The model under review builds one solid part; all positions refer to its coordinate system, in mm. A direction names the side the tool comes from. Coordinates: 2 decimals unless noted, no trailing zeros. Write each loop counter-clockwise with the first axis right and the second up, starting at its lowest first coordinate (ties: lowest second). Pieces come first, ordered by that corner, then holes.
1) Add section A-A, the plane x = 16.5. State the section outline as (y, z) points.
2) For P1, Ø1.5, axis at y = 152.5, z = -1, coming from the -X side; P2, Ø1, axis at x = -19, z = -7, coming from the -Y side; P3, Ø0.8, axis at y = 135.5, z = -0.5, coming from the +X side; P4, Ø2.5, axis at x = -24.73, y = 109, coming from the +Z side, all flat-tipped, find the tip position at first contact; note any pin that passes through.
3) Add section C-C, the plane z = -6.25. State the section outline as (x, y) points, then the cut area to 3 significant figures.
4) Add section B-B, the plane y = 44.5. State the section outline as (x, z) points, then the cut area to 3 significant figures.
5) For line 1 (Z direction, x = 31.5, y = 92.5); line 2 (X direction, y = 22, z = -0.25); line 3 (Y direction, x = 29, z = -0.7), list the stretches that pass through material, from the lowest coordinate up.
6) Machinability: for faces 5 (the flat face through (-1, 97, -1)), 6 (the flat face through (35.323, 86.552, -0.493)), 7 (the flat face through (1, 213, -8.485)), 8 (the flat face through (-35.177, 87.448, -0.493)), which of the approach directions +Z, -Z, +X, -X, +Y, -Y give a long, thin tool a straight path to every point of the face, cutting with its end or side? Answer none if there is none.
7) Mouldability with a two-part tool opening along Y and no side actions: class faces 1 (the cylindrical face through (46.996, 159.626, -0.493)), 2 (the flat face through (-1, 97, 0)), 3 (the cylindrical face through (-46.996, 160.374, -0.493)), 4 (the flat face through (-0.42, 196.749, -4.335)) as released by +Y, released by -Y, zero draft, split by the parting line, or undercut.
from build123d import *

# Parameters (mm, degrees)
BASE_FLANGE1_DEPTH           = 1
EDGE_FLANGE1_STRIP_CUT_DEPTH = 60
EDGE_FLANGE1_DEPTH           = 60
EDGE_FLANGE2_STRIP_CUT_DEPTH = 60
EDGE_FLANGE2_DEPTH           = 60
SKETCH14_W                   = 1
SKETCH14_H                   = 24.280676727
BOSS_EXTRUDE1_DEPTH          = 9
SKETCH15_W                   = 1
SKETCH15_H                   = 24.280676727
BOSS_EXTRUDE2_DEPTH          = 9
CUT_EXTRUDE1_START           = -1
CUT_EXTRUDE1_DEPTH           = 1
FILLET2_R                    = 2
SKETCH17_R                   = 1.5
CUT_EXTRUDE2_DEPTH           = 231.487770095
SKETCH18_R                   = 1.5
CUT_EXTRUDE3_DEPTH           = 231.487770095
SKETCH19_R                   = 1.5
CUT_EXTRUDE4_DEPTH           = 231.487770095


# Read off the part's stored shape, not the designer's step: Cut-Extrude1
# Sheet-metal steps are written as plain solids
with BuildPart() as part:
    # Sketch1 → Base-Flange1 (new body)
    with BuildSketch(Plane.XY):
        with BuildLine():
            Line((-40.5, 0), (40.5, 0))
            Line((40.5, 0), (40.5, 55))
            Line((40.5, 55), (30, 119))
            Line((30, 119), (30, 143))
            ThreePointArc((30, 143), (47, 160), (30, 177))
            Line((30, 177), (30, 192))
            Line((30, 192), (-30, 192))
            Line((-30, 192), (-30, 177))
            ThreePointArc((-30, 177), (-47, 160), (-30, 143))
            Line((-30, 143), (-30, 119))
            Line((-30, 119), (-40.5, 55))
            Line((-40.5, 55), (-40.5, 0))
        make_face()
    extrude(amount=-BASE_FLANGE1_DEPTH)

    # Edge-Flange1 strip (across the edge) → Edge-Flange1 strip cut (cut)
    with BuildSketch(Plane(origin=(-30, 192, -1), x_dir=(0, -0.7071067811865438, -0.7071067811865512), z_dir=(1, 0, 0))):
        Polygon((-4.361498471, 2.947284909), (-0.491361636, -0.922851926), (0.215745145, -0.215745145), (-3.65439169, 3.65439169), align=None)
    extrude(amount=EDGE_FLANGE1_STRIP_CUT_DEPTH, mode=Mode.SUBTRACT)

    # Edge-Flange1 section (across the edge) → Edge-Flange1 (add)
    with BuildSketch(Plane(origin=(-30, 192, -1), x_dir=(0, -0.7071067811865438, -0.7071067811865512), z_dir=(1, 0, 0))):
        with BuildLine():
            Line((-1, 0.30510971), (-1, 11.585786438))
            Line((-1, 11.585786438), (0, 11.585786438))
            Line((0, 11.585786438), (0, 0.30510971))
            ThreePointArc((0, 0.30510971), (0.056070336, 0.023225094), (0.215745145, -0.215745145))
            Line((0.215745145, -0.215745145), (-0.491361636, -0.922851926))
            ThreePointArc((-0.491361636, -0.922851926), (-0.867809196, -0.359458339), (-1, 0.30510971))
        make_face()
    extrude(amount=EDGE_FLANGE1_DEPTH)

    # Edge-Flange2 strip (across the edge) → Edge-Flange2 strip cut (cut)
    with BuildSketch(Plane(origin=(30, 200.899494937, -8.485281374), x_dir=(0, 0, 1), z_dir=(-1, 0, 0))):
        Polygon((-4.361498471, 2.947284909), (-0.491361636, -0.922851926), (0.215745145, -0.215745145), (-3.65439169, 3.65439169), align=None)
    extrude(amount=EDGE_FLANGE2_STRIP_CUT_DEPTH, mode=Mode.SUBTRACT)

    # Edge-Flange2 section (across the edge) → Edge-Flange2 (add)
    with BuildSketch(Plane(origin=(30, 200.899494937, -8.485281374), x_dir=(0, 0, 1), z_dir=(-1, 0, 0))):
        with BuildLine():
            Line((-1, 0.30510971), (-1, 24.585786438))
            Line((-1, 24.585786438), (0, 24.585786438))
            Line((0, 24.585786438), (0, 0.30510971))
            ThreePointArc((0, 0.30510971), (0.056070336, 0.023225094), (0.215745145, -0.215745145))
            Line((0.215745145, -0.215745145), (-0.491361636, -0.922851926))
            ThreePointArc((-0.491361636, -0.922851926), (-0.867809196, -0.359458339), (-1, 0.30510971))
        make_face()
    extrude(amount=EDGE_FLANGE2_DEPTH)

    # Sketch14 → Boss-Extrude1 (add)
    with BuildSketch(Plane(origin=(30, 0, 0), x_dir=(0, 0, -1), z_dir=(1, 0, 0))):
        with Locations((8.985281374, 213.344943011)):
            Rectangle(SKETCH14_W, SKETCH14_H)
    extrude(amount=BOSS_EXTRUDE1_DEPTH)

    # Sketch15 → Boss-Extrude2 (add)
    with BuildSketch(Plane.ZY.offset(30)):
        with Locations((-8.985281374, 213.344943011)):
            Rectangle(SKETCH15_W, SKETCH15_H)
    extrude(amount=BOSS_EXTRUDE2_DEPTH)

    # Cut-Extrude1 outline → Cut-Extrude1 (cut)
    with BuildSketch(Plane(origin=(0, 0, -9.485281374), x_dir=(-1, 0, 0), z_dir=(0, 0, -1)).offset(CUT_EXTRUDE1_START)):
        with BuildLine():
            Line((39, 201.204604647), (39, 219.240417061))
            add(Edge.make_bspline(
                [(30, 201.204604647), (31.71398357, 204.270148777), (35.194685688, 209.766177292), (38.784446875, 217.082662856), (39, 219.240417061)],
                knots=[0, 0, 0, 0, 0.463591524, 0.691545034, 0.691545034, 0.691545034, 0.691545034], degree=3))
            Line((30, 201.204604647), (39, 201.204604647))
        make_face()
        with BuildLine():
            add(Edge.make_bspline(
                [(39, 220.550582239), (38.73699137, 222.877809464), (36.937902842, 224.748781209), (32.132158029, 225.485281374)],
                knots=[0.73898762, 0.73898762, 0.73898762, 0.73898762, 1, 1, 1, 1], degree=3))
            Line((39, 220.550582239), (39, 225.485281374))
            Line((39, 225.485281374), (32.132158029, 225.485281374))
        make_face()
    cut_extrude1 = extrude(amount=CUT_EXTRUDE1_DEPTH, mode=Mode.SUBTRACT)

    # Mirror1: Cut-Extrude1 across plane
    add(cut_extrude1.mirror(Plane(origin=(0, 0, 0), x_dir=(0, 0, 1), z_dir=(1, 0, 0))), mode=Mode.SUBTRACT)

    # Fillet2
    fillet2_edges = [part.edges().sort_by_distance(p)[0] for p in [
        (40.5, 0, -0.5),
        (-40.5, 0, -0.5),
    ]]
    fillet(fillet2_edges, radius=FILLET2_R)

    # Sketch17 → Cut-Extrude2 (cut, through all)
    with BuildSketch(Plane(origin=(0, 0, -1), x_dir=(-1, 0, 0), z_dir=(0, 0, -1))):
        with Locations((-35.5, 5)):
            Circle(SKETCH17_R)
        with Locations((35.5, 5)):
            Circle(SKETCH17_R)
        with Locations((-35.5, 55)):
            Circle(SKETCH17_R)
        with Locations((35.5, 55)):
            Circle(SKETCH17_R)
    extrude(amount=-CUT_EXTRUDE2_DEPTH, mode=Mode.SUBTRACT)

    # Sketch18 → Cut-Extrude3 (cut, through all)
    with BuildSketch(Plane(origin=(0, 0, -1), x_dir=(-1, 0, 0), z_dir=(0, 0, -1))):
        with Locations((-29, 67)):
            Circle(SKETCH18_R)
        with Locations((29, 67)):
            Circle(SKETCH18_R)
        with Locations((-25.274058899, 109)):
            Circle(SKETCH18_R)
        with Locations((24.725941101, 109)):
            Circle(SKETCH18_R)
    extrude(amount=-CUT_EXTRUDE3_DEPTH, mode=Mode.SUBTRACT)

    # Sketch19 → Cut-Extrude4 (cut, through all)
    with BuildSketch(Plane(origin=(0, 0, -1), x_dir=(-1, 0, 0), z_dir=(0, 0, -1))):
        with Locations((-32, 160)):
            Circle(SKETCH19_R)
        with Locations((32, 160)):
            Circle(SKETCH19_R)
        with Locations((-32, 150)):
            Circle(SKETCH19_R)
        with Locations((32, 150)):
            Circle(SKETCH19_R)
    extrude(amount=-CUT_EXTRUDE4_DEPTH, mode=Mode.SUBTRACT)


solid = part.part
Geometry results:
1. outline: (0, -1) - (191.69, -1) arc R0.74 cw to (192.22, -1.22) - (199.98, -8.98) arc R1.74 ccw to (201.2, -9.49) - (225.49, -9.49) - (225.49, -8.49) - (201.2, -8.49) arc R0.74 cw to (200.68, -8.27) - (192.92, -0.51) arc R1.74 ccw to (191.69, 0) - (0, 0) - close
2. P1: stops at x = -45.6
2. P2: stops at y = 197.5
2. P3: stops at x = 30
2. P4: passes through
3. outline: (-30, 197.25) - (30, 197.25) - (30, 198.66) - (-30, 198.66) - close
3. area: 84.9 mm2
4. outline: (-40.5, -1) - (40.5, -1) - (40.5, 0) - (-40.5, 0) - close
4. area: 81.0 mm2
5. line 1: z = -1 to 0
5. line 2: x = -40.5 to 40.5
5. line 3: y = 0 to 65.5, 68.5 to 193.11
6. face 5: -Z, +X, -X, -Y
6. face 6: +Z, -Z, +X
6. face 7: +Z, +X, -X, +Y
6. face 8: +Z, -Z, -X
7. face 1: undercut
7. face 2: zero draft
7. face 3: undercut
7. face 4: released by +Y
